```python
from build123d import *

# Parameters (mm, degrees)
SKETCH1_R               = 1.75
SKETCH1_W               = 7.2
SKETCH1_H               = 10.8
BOSS_EXTRUDE2_DEPTH     = 5
FILLET1_R               = 5.4
FILLET2_R               = 5.4
FILLET3_RADIUS          = 10
FILLET3_LENGTH          = 5
SKETCH2_W               = 35
SKETCH2_H               = 19.782608696
SKETCH2_W_2             = 23
SKETCH2_H_2             = 13
BOSS_EXTRUDE3_DEPTH     = 5.5
SKETCH3_W               = 23
SKETCH3_H               = 13
CUT_EXTRUDE1_DEPTH      = 3.5
CUT_EXTRUDE2_DEPTH      = 76.201396264
CUT_EXTRUDE2_DEPTH_BACK = 76.201396264
SKETCH6_W               = 13.4
SKETCH6_H               = 0.108695652
CUT_EXTRUDE3_DEPTH      = 13.5
SKETCH7_W               = 8
SKETCH7_H               = 28
BOSS_EXTRUDE5_DEPTH     = 38
SKETCH8_R               = 2.5
CUT_EXTRUDE4_DEPTH      = 32
FILLET5_R               = 10
SKETCH9_R               = 1
CUT_EXTRUDE5_DEPTH      = 7
BOSS_EXTRUDE6_START     = -8
BOSS_EXTRUDE6_DEPTH     = 8
CUT_EXTRUDE8_DEPTH      = 97.444595494
FILLET8_R               = 8
FILLET10_R              = 4
BOSS_EXTRUDE7_START     = -1.5
BOSS_EXTRUDE7_OUTLINE_W = 23
BOSS_EXTRUDE7_OUTLINE_H = 13
BOSS_EXTRUDE7_DEPTH     = 1.5
SKETCH15_R              = 1
BOSS_EXTRUDE8_DEPTH     = 7
SKETCH16_W              = 23
SKETCH16_H              = 13
BOSS_EXTRUDE9_DEPTH     = 9
SKETCH23_W              = 22.4
SKETCH23_H              = 19.782608696
BOSS_EXTRUDE11_DEPTH    = 10.5
SKETCH32_W              = 2
SKETCH32_H              = 19.782608696
CUT_EXTRUDE10_DEPTH     = 112.132758447
SKETCH33_W              = 21.6
SKETCH33_H              = 4.008695652
BOSS_EXTRUDE26_DEPTH    = 5.5
SKETCH34_W              = 33.8
SKETCH34_H              = 4.008695652
BOSS_EXTRUDE27_DEPTH    = 10.5
SKETCH39_W              = 41.4
SKETCH39_H              = 21
CUT_EXTRUDE15_DEPTH     = 6
SKETCH40_R              = 1
CUT_EXTRUDE16_DEPTH     = 7
SKETCH41_R              = 1.75
SKETCH41_R_2            = 3.75
CUT_EXTRUDE17_DEPTH     = 111.965264835
CUT_EXTRUDE18_DEPTH     = 10
FILLET12_R              = 5
BOSS_EXTRUDE28_REACH    = 109.184


with BuildPart() as part:
    # Sketch1 → Boss-Extrude2 (new body)
    # profile 1 of 2: a face of its own
    with BuildSketch(Plane(origin=(0, 0, 0), x_dir=(1, 0, 0), z_dir=(0, 1, 0))):
        Polygon((26, 45), (10, 45), (0, 33.819660113), (0, 15), (10, 0), (26, 0), (36, 15), (60, 15), (60, 35), (36, 35), align=None)
        with Locations(Location((13, 5, 0), (0, 0, 270))):
            Circle(SKETCH1_R, mode=Mode.SUBTRACT)
        with Locations(Location((23, 5, 0), (0, 0, 270))):
            Circle(SKETCH1_R, mode=Mode.SUBTRACT)
        with Locations(Location((5, 25, 0), (0, 0, 270))):
            Circle(SKETCH1_R, mode=Mode.SUBTRACT)
        Polygon((26.5, 30.4), (37.3, 30.4), (44.5, 30.4), (44.5, 19.6), (37.3, 19.6), (26.5, 19.6), align=None, mode=Mode.SUBTRACT)
    # profile 2 of 2: a face of its own
    with BuildSketch(Plane(origin=(0, 0, 0), x_dir=(1, 0, 0), z_dir=(0, 1, 0))):
        with Locations((40.9, 25)):
            Rectangle(SKETCH1_W, SKETCH1_H)
    extrude(amount=BOSS_EXTRUDE2_DEPTH)

    # Fillet1
    fillet1_edges = [part.edges().sort_by_distance(p)[0] for p in [
        (37.3, 2.5, -19.6),
        (37.3, 2.5, -30.4),
    ]]
    fillet(fillet1_edges, radius=FILLET1_R - 0.0001)  # a hair under: the kernel refuses the full size

    # Fillet2
    fillet2_edges = [part.edges().sort_by_distance(p)[0] for p in [
        (26.5, 2.5, -30.4),
        (26.5, 2.5, -19.6),
    ]]
    fillet(fillet2_edges, radius=FILLET2_R - 0.0001)  # a hair under: the kernel refuses the full size

    # Fillet3: full round fillet: the end face becomes a half cylinder, R = half its width
    fillet3_face = Plane((60, 2.5, -25), x_dir=(0, 1, 0), z_dir=(1, 0, 0))  # on the end face: x along it, z out of the body
    fillet3_slab = fillet3_face.offset(-FILLET3_RADIUS / 2) * Box(FILLET3_LENGTH, 2 * FILLET3_RADIUS, FILLET3_RADIUS, mode=Mode.PRIVATE)  # the body's end, R deep
    fillet3_round = Plane((50, 2.5, -25), x_dir=(1, 0, 0), z_dir=(0, 1, 0)) * Cylinder(FILLET3_RADIUS, FILLET3_LENGTH, mode=Mode.PRIVATE)  # its axis R under the face
    add(fillet3_slab - fillet3_round, mode=Mode.SUBTRACT)

    # Sketch2 → Boss-Extrude3 (add)
    with BuildSketch(Plane.XZ):
        with Locations((31.9, -25)):
            Rectangle(SKETCH2_W, SKETCH2_H)
        with Locations((31.9, -25)):
            Rectangle(SKETCH2_W_2, SKETCH2_H_2, mode=Mode.SUBTRACT)
    extrude(amount=BOSS_EXTRUDE3_DEPTH)

    # Sketch3 → Cut-Extrude1 (cut)
    with BuildSketch(Plane.XZ):
        with Locations((31.9, -25)):
            Rectangle(SKETCH3_W, SKETCH3_H)
    extrude(amount=-CUT_EXTRUDE1_DEPTH, mode=Mode.SUBTRACT)

    # Sketch4 → Cut-Extrude2 (cut, two sides: drawn at the far end of the back side and taken through both)
    with BuildSketch(Plane.XZ.offset(-CUT_EXTRUDE2_DEPTH_BACK)):
        with BuildLine():
            Line((49.4, -15), (49.4, -35))
            Line((49.4, -35), (50, -35))
            ThreePointArc((50, -35), (60, -25), (50, -15))
            Line((50, -15), (49.4, -15))
        make_face()
    extrude(amount=CUT_EXTRUDE2_DEPTH + CUT_EXTRUDE2_DEPTH_BACK, mode=Mode.SUBTRACT)

    # Sketch6 → Cut-Extrude3 (cut)
    with BuildSketch(Plane.XZ):
        with Locations((42.7, -34.945652174)):
            Rectangle(SKETCH6_W, SKETCH6_H)
        with Locations((42.7, -15.054347826)):
            Rectangle(SKETCH6_W, SKETCH6_H)
    extrude(amount=-CUT_EXTRUDE3_DEPTH, mode=Mode.SUBTRACT)

    # Sketch7 → Boss-Extrude5 (add)
    with BuildSketch(Plane(origin=(0, 0, -45), x_dir=(-1, 0, 0), z_dir=(0, 0, -1))):
        with Locations((-10, -9)):
            Rectangle(SKETCH7_W, SKETCH7_H)
    extrude(amount=BOSS_EXTRUDE5_DEPTH)

    # Sketch8 → Cut-Extrude4 (cut)
    with BuildSketch(Plane(origin=(14, 0, 0), x_dir=(0, 0, -1), z_dir=(1, 0, 0))):
        with Locations(Location((69, -9, 0), (0, 0, 90))):
            Circle(SKETCH8_R)
    extrude(amount=-CUT_EXTRUDE4_DEPTH, mode=Mode.SUBTRACT)

    # Fillet5
    fillet5_edges = [part.edges().sort_by_distance(p)[0] for p in [
        (10, -23, -83),
        (10, 5, -83),
    ]]
    fillet(fillet5_edges, radius=FILLET5_R)

    # Sketch9 → Cut-Extrude5 (cut)
    with BuildSketch(Plane.XZ.offset(5.5)):
        with Locations(Location((18.1, -25, 0), (0, 0, 270))):
            Circle(SKETCH9_R)
        with Locations(Location((45.7, -25, 0), (0, 0, 270))):
            Circle(SKETCH9_R)
    extrude(amount=-CUT_EXTRUDE5_DEPTH, mode=Mode.SUBTRACT)

    # Sketch10 → Boss-Extrude6 (add)
    with BuildSketch(Plane.ZY.offset(-6).offset(BOSS_EXTRUDE6_START)):
        Polygon((-45, -23), (-45, 5), (-34.891304348, 5), (-34.891304348, -5.5), align=None)
    extrude(amount=BOSS_EXTRUDE6_DEPTH)

    # Sketch13 → Cut-Extrude8 (cut, through all)
    with BuildSketch(Plane.ZY.offset(-6)):
        Polygon((-45, -23), (-34.891304348, -5.5), (-55, -23), align=None)
    extrude(amount=-CUT_EXTRUDE8_DEPTH, mode=Mode.SUBTRACT)

    # Fillet8
    fillet8_edges = [part.edges().sort_by_distance(p)[0] for p in [
        (10, -5.5, -34.891304348),
        (10, -23, -55),
    ]]
    fillet(fillet8_edges, radius=FILLET8_R)

    # Fillet10
    fillet10_edges = [part.edges().sort_by_distance(p)[0] for p in [
        (14, -9, -83),
        (14, -23, -65.496815266),
        (14, 5, -59),
        (14, -20.071067812, -80.071067812),
        (14, 2.071067812, -80.071067812),
        (14, -14.463184152, -45.19061533),
        (14, -0.928447255, -34.891304348),
        (14, -22.492592848, -55.189873693),
        (14, -5.172402248, -35.610685663),
    ]]
    fillet(fillet10_edges, radius=FILLET10_R)

    # Boss-Extrude7: read off the stored shape, not the designer's step
    # Boss-Extrude7 outline → Boss-Extrude7 (add)
    with BuildSketch(Plane.XZ.offset(-3.5).offset(BOSS_EXTRUDE7_START)):
        with Locations((31.9, -25)):
            Rectangle(BOSS_EXTRUDE7_OUTLINE_W, BOSS_EXTRUDE7_OUTLINE_H)
    extrude(amount=BOSS_EXTRUDE7_DEPTH)

    # Sketch15 → Boss-Extrude8 (add)
    with BuildSketch(Plane.XZ.offset(5.5)):
        with Locations((18.1, -25)):
            Circle(SKETCH15_R)
        with Locations((45.7, -25)):
            Circle(SKETCH15_R)
    extrude(amount=-BOSS_EXTRUDE8_DEPTH)

    # Sketch16 → Boss-Extrude9 (add)
    with BuildSketch(Plane.XZ.offset(-3.5)):
        with Locations((31.9, -25)):
            Rectangle(SKETCH16_W, SKETCH16_H)
    extrude(amount=BOSS_EXTRUDE9_DEPTH)

    # Sketch23 → Boss-Extrude11 (add)
    with BuildSketch(Plane.XZ.offset(5.5)):
        with Locations((60.6, -25)):
            Rectangle(SKETCH23_W, SKETCH23_H)
    extrude(amount=-BOSS_EXTRUDE11_DEPTH)

    # Sketch32 → Cut-Extrude10 (cut, through all)
    with BuildSketch(Plane.XZ.offset(5.5)):
        with Locations((70.8, -25)):
            Rectangle(SKETCH32_W, SKETCH32_H)
    extrude(amount=-CUT_EXTRUDE10_DEPTH, mode=Mode.SUBTRACT)

    # Sketch33 → Boss-Extrude26 (add)
    with BuildSketch(Plane.XZ.offset(5.5)):
        with Locations((25.2, -13.104347826)):
            Rectangle(SKETCH33_W, SKETCH33_H)
        with Locations((25.2, -36.895652174)):
            Rectangle(SKETCH33_W, SKETCH33_H)
    extrude(amount=-BOSS_EXTRUDE26_DEPTH)

    # Sketch34 → Boss-Extrude27 (add)
    with BuildSketch(Plane.XZ.offset(5.5)):
        with Locations((52.9, -13.104347826)):
            Rectangle(SKETCH34_W, SKETCH34_H)
        with Locations((52.9, -36.895652174)):
            Rectangle(SKETCH34_W, SKETCH34_H)
    extrude(amount=-BOSS_EXTRUDE27_DEPTH)

    # Sketch39 → Cut-Extrude15 (cut)
    with BuildSketch(Plane.XZ.offset(5.5)):
        with Locations((42.1, -25)):
            Rectangle(SKETCH39_W, SKETCH39_H)
    extrude(amount=-CUT_EXTRUDE15_DEPTH, mode=Mode.SUBTRACT)

    # Sketch40 → Cut-Extrude16 (cut)
    with BuildSketch(Plane.XZ.offset(5.5)):
        with Locations(Location((66.35, -30, 0), (0, 0, 270))):
            Circle(SKETCH40_R)
        with Locations(Location((66.35, -20, 0), (0, 0, 270))):
            Circle(SKETCH40_R)
        with Locations(Location((17.85, -30, 0), (0, 0, 270))):
            Circle(SKETCH40_R)
        with Locations(Location((17.85, -20, 0), (0, 0, 270))):
            Circle(SKETCH40_R)
    extrude(amount=-CUT_EXTRUDE16_DEPTH, mode=Mode.SUBTRACT)

    # Sketch41 → Cut-Extrude17 (cut, through all)
    with BuildSketch(Plane.XZ.offset(-0.5)):
        with Locations(Location((5, -25, 0), (0, 0, 90))):
            Circle(SKETCH41_R)
        with Locations(Location((31.9, -25, 0), (0, 0, 270))):
            Circle(SKETCH41_R_2)
    extrude(amount=-CUT_EXTRUDE17_DEPTH, mode=Mode.SUBTRACT)

    # Sketch42 → Cut-Extrude18 (cut)
    with BuildSketch(Plane(origin=(0, 0, 0), x_dir=(1, 0, 0), z_dir=(0, 1, 0))):
        Polygon((14, 45), (14, 38.891304348), (32.1, 38.9), (26, 45), align=None)
    extrude(amount=CUT_EXTRUDE18_DEPTH, mode=Mode.SUBTRACT)

    # Fillet12
    fillet12_edges = [part.edges().sort_by_distance(p)[0] for p in [
        (69.8, -0.25, -11.1),
        (69.8, -0.25, -38.9),
    ]]
    fillet(fillet12_edges, radius=FILLET12_R)

    # Boss-Extrude28: up to this face of the body (flat: up to its plane)
    boss_extrude28_end = Plane(part.part.faces().sort_by_distance((14.4, -2.75, -25))[0])
    # Sketch44 → Boss-Extrude28 (add, up to the picked face)
    with BuildSketch(Plane.ZY.offset(-6), mode=Mode.PRIVATE) as boss_extrude28_sk1:
        Polygon((-40.527864045, 0), (-34.78782211, 0), (-35.237020655, -4.368087235), (-35.768960465, -5.5), (-40.049862217, -5.5), align=None)
    boss_extrude28_tool1 = split(extrude(boss_extrude28_sk1.sketch, amount=-BOSS_EXTRUDE28_REACH, mode=Mode.PRIVATE), bisect_by=boss_extrude28_end, keep=Keep.BOTH, mode=Mode.PRIVATE)
    add(boss_extrude28_tool1.solids().sort_by(Axis((6, -2.637977, -37.697403), (1, 0, 0)))[0])


solid = part.part
```
Work out the finished part from the listing and answer in its coordinate system (mm). A direction names the side the tool comes from. Give positions to 0.01 mm unless a question says otherwise; leave off trailing zeros. Loops run counter-clockwise (first coordinate to the right, second up) from the corner with the lowest first, then second, coordinate; pieces in that order, holes last. Notation, with made-up numbers: (29, -19.5) -> (47, -19.5) arc R30 ccw to (47, 16.5) -> close; hole circle Ø6 at (63.25, 70). An arc over 180 degrees is marked (long way). Put each result on its own line as item: value. Start each with the question number.
Item 1: The part is cut by section B-B (z = -24.5). Give the vertices of the cut face in (x, y).
Item 2: The part is cut by section A-A (x = 9). Give the vertices of the cut face in (y, z), then the cut area to 3 significant figures.
Item 3: Each of these flat-tipped pins is pushed along its axis until it touches: P1, Ø5, axis at y = -10, z = -37, coming from the +X side; P2, Ø1, axis at x = 17.5, z = -30, coming from the -Y side; P3, Ø2, axis at x = 66.5, z = -30, coming from the -Y side; P4, Ø3.5, axis at x = 34, z = -37.5, coming from the +Y side. Where does it stop, or does it pass through?
Item 4: The mould has two halves that part along Z. Classify faces 4 (the face through (66, 1.5, -30)), 5 (the face through (4.93, 2.465, -7.605)), 6 (the face through (0, 2, -25)), 7 (the face through (45, -1, -38.9)): released by +Z, released by -Z, zero draft, split by the parting line, or undercut.
Item 5: Which of the six approach directions +Z, -Z, +X, -X, +Y, -Y give full straight-line access (tool end or side, diameter ignored) to faces 1 (the face through (13, 0, -16)), 2 (the face through (21.4, -3, -25)), 3 (the face through (11.07, -1.67, -34.96))?
Item 6: The part is cut by section C-C (x = 53). Give the vertices of the cut face in (y, z).
Item 7: Find the intervals of material crossed by L1, parallel to X at y = -3.75, z = -30; L2, parallel to X at y = 4.15, z = -25; L3, parallel to Z at x = 23, y = -2.75, in increasing order. Write a range as [from, to].
Answers below:
1. outline: (0, 0) -> (3.32, 0) -> (3.32, 5) -> (0, 5) -> close; (6.68, 0) -> (14.4, 0) -> (14.4, -5.5) -> (21.4, -5.5) -> (21.4, 0.5) -> (28.18, 0.5) -> (28.18, 5) -> (6.68, 5) -> close; (35.62, 0.5) -> (62.8, 0.5) -> (62.8, -5.5) -> (69.8, -5.5) -> (69.8, 5) -> (35.62, 5) -> close
2. outline: (-23, -73) arc R10 ccw to (-13, -83) -> (-5, -83) arc R10 ccw to (5, -73) -> (5, -1.5) -> (0, -1.5) -> (0, -34.79) -> (-1.01, -34.89) -> (-1.86, -34.89) arc R8 ccw to (-4.09, -35.21) -> (-4.37, -35.24) -> (-5.02, -35.54) arc R8 ccw to (-7.89, -37.64) -> (-21.03, -52.74) arc R8 ccw to (-23, -57.99) -> close; hole circle Ø5 at (-9, -69)
2. area: 1,270 mm2
3. P1: x = 11.92
3. P2: y = 1.5
3. P3: y = -5.5
3. P4: y = 5
4. face 4: undercut
4. face 5: released by +Z
4. face 6: zero draft
4. face 7: released by -Z
5. face 1: +Z, -X, -Y
5. face 2: -Y
5. face 3: +Z, -Y
6. outline: (-5.5, -38.9) -> (5, -38.9) -> (5, -11.1) -> (-5.5, -11.1) -> (-5.5, -14.5) -> (0.5, -14.5) -> (0.5, -35.5) -> (-5.5, -35.5) -> close
7. L1: [14.4, 16.85], [18.85, 21.4], [62.8, 65.35], [67.35, 69.8]
7. L2: [0, 3.25], [6.75, 28.15], [35.65, 69.8]
7. L3: [-38.9, -35.5], [-14.5, -11.1]
